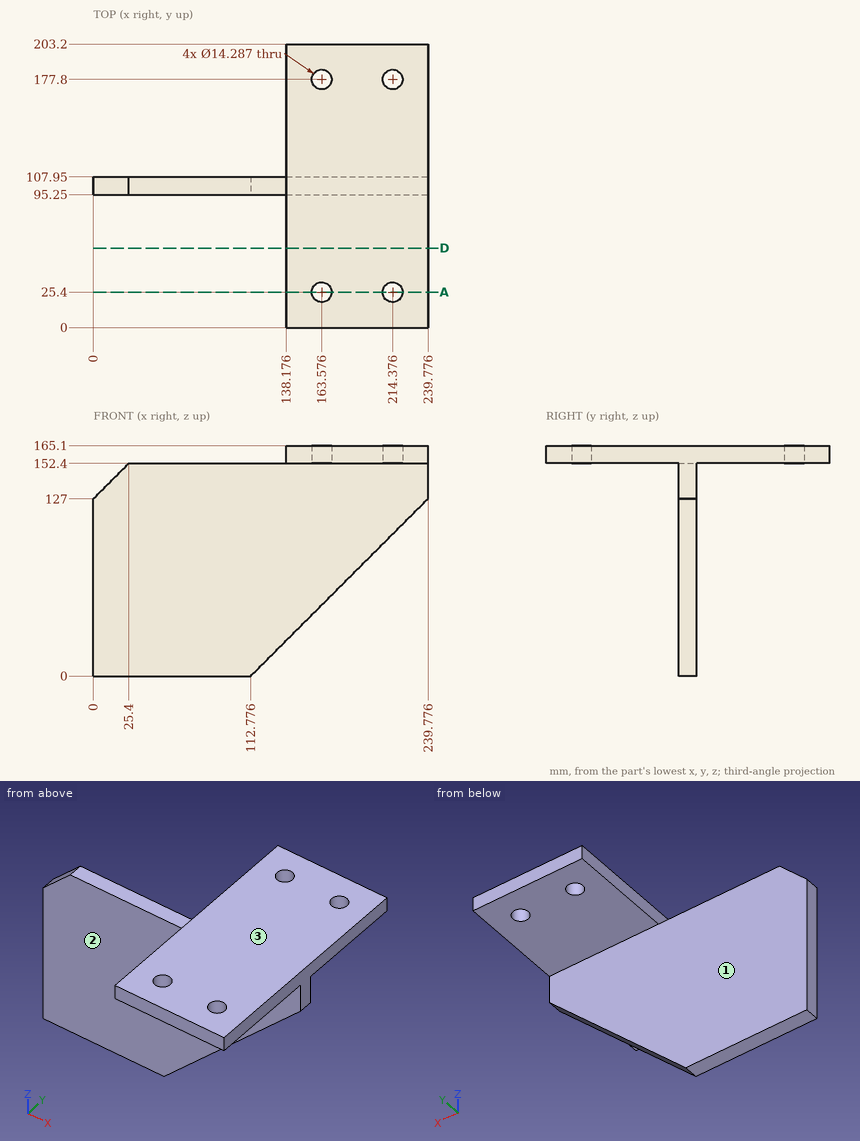
Study the drawing (mm; zero at the part's minimum x, y, z) and answer. A direction names the side the tool comes from. Give positions to 0.01 mm unless a question says otherwise; leave off trailing zeros. Write each loop counter-clockwise with the first axis right and the second up, starting at its lowest first coordinate (ties: lowest second). Pieces come first, ordered by that corner, then holes. Notation, with made-up numbers: M 58,-8.75 L 62,-8.75 A28 cw 62,29.25 Z; hole C 23.25,49.5 d9. An arc over 180 degrees is marked long. Put each result on its own line as item: value. Start each with the question number.
1. Which of the six approach directions +Z, -Z, +X, -X, +Y, -Y give full straight-line access (tool end or side, diameter ignored) to the marked faces 1, 2 and 3?
2. Consider line 1 along X through (y, z) = (25, 156) (1 decimal); line 2 along Y through (x, z) = (77.5, 55.5); line 3 along Z through (x, y) = (176, 150.5). Determine where each line is inside the solid, lowest interval first.
3. Each of these flat-tipped pins is pushed along its axis until it touches: pin 1 Ø13 at (x, y) = (214.376, 25.4) entering from -Z; pin 2 Ø14 at (y, z) = (78.5, 156.5) entering from -X; pin 3 Ø12 at (x, z) = (80.5, 134.5) entering from -Y; pin 4 Ø4 at (x, y) = (54, 104.5) entering from +Z. Where does it stop, or does it pass through?
4. The part is cut by section A-A, the plane y = 25.4. Give the vertices of the cut face in (x, z) (1 decimal).
5. The part is cut by section D-D, the plane y = 57. Give the vertices of the cut face in (x, z) (1 decimal).
Final values:
1. face 1: -Z, +X, -X, +Y
1. face 2: -Z, +X, -X, -Y
1. face 3: +Z, +X, -X, +Y, -Y
2. line 1: x = 138.2 to 156.4, 170.7 to 207.2, 221.5 to 239.8
2. line 2: y = 95.25 to 107.95
2. line 3: z = 152.4 to 165.1
3. pin 1: passes through
3. pin 2: stops at x = 138.18
3. pin 3: stops at y = 95.25
3. pin 4: stops at z = 152.4
4. outline: M 138.2,152.4 L 156.4,152.4 L 156.4,165.1 L 138.2,165.1 Z; M 170.7,152.4 L 207.2,152.4 L 207.2,165.1 L 170.7,165.1 Z; M 221.5,152.4 L 239.8,152.4 L 239.8,165.1 L 221.5,165.1 Z
5. outline: M 138.2,152.4 L 239.8,152.4 L 239.8,165.1 L 138.2,165.1 Z
